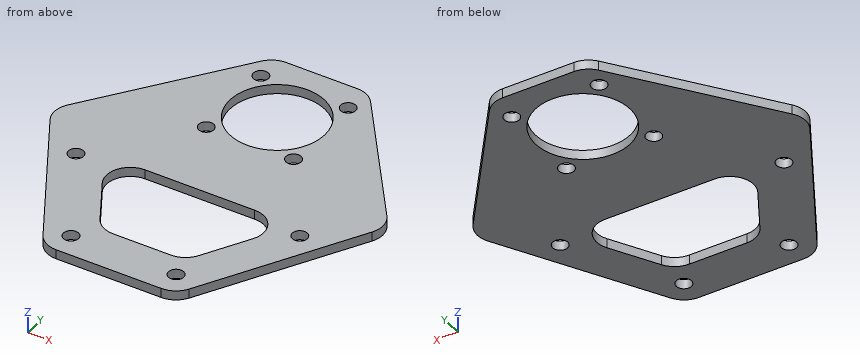
```python
from build123d import *

# Parameters (mm, degrees)
EXTRUDE_1_OUTLINE_R   = 1.6
EXTRUDE_1_OUTLINE_R_2 = 10
EXTRUDE_1_DEPTH       = 2
FILLET_1_R            = 5


# Read off the part's stored shape, not the designer's step: ﾎﾞｽ - 押し出し1
with BuildPart() as part:
    # ﾎﾞｽ - 押し出し1 outline → ﾎﾞｽ - 押し出し1 (new body)
    with BuildSketch(Plane.XY):
        Polygon((-15.011106999, -35), (12.897858345, -35), (34.473029949, 2.369293401), (10, 35), (-10, 35), (-35.667090423, 0.77721277), align=None)
        with Locations((-12.124355653, -30)):
            Circle(EXTRUDE_1_OUTLINE_R, mode=Mode.SUBTRACT)
        with Locations((-24.624355653, -8.349364905)):
            Circle(EXTRUDE_1_OUTLINE_R, mode=Mode.SUBTRACT)
        with Locations((10.011106999, -30)):
            Circle(EXTRUDE_1_OUTLINE_R, mode=Mode.SUBTRACT)
        with BuildLine():
            Line((6.062177826, -25.5), (-6.062177826, -25.5))
            ThreePointArc((-6.062177826, -25.5), (-8.562177826, -24.830127019), (-10.392304845, -23))
            Line((-10.392304845, -23), (-15.877132403, -13.5))
            ThreePointArc((-15.877132403, -13.5), (-15.877132403, -8.5), (-11.547005384, -6))
            Line((-11.547005384, -6), (11.547005384, -6))
            ThreePointArc((11.547005384, -6), (15.877132403, -8.5), (15.877132403, -13.5))
            Line((15.877132403, -13.5), (10.392304845, -23))
            ThreePointArc((10.392304845, -23), (8.562177826, -24.830127019), (6.062177826, -25.5))
        make_face(mode=Mode.SUBTRACT)
        with Locations((22.511106999, -8.349364905)):
            Circle(EXTRUDE_1_OUTLINE_R, mode=Mode.SUBTRACT)
        with Locations((-9.192388155, 10.807611845)):
            Circle(EXTRUDE_1_OUTLINE_R, mode=Mode.SUBTRACT)
        with Locations((-9.192388155, 29.192388155)):
            Circle(EXTRUDE_1_OUTLINE_R, mode=Mode.SUBTRACT)
        with Locations((9.192388155, 10.807611845)):
            Circle(EXTRUDE_1_OUTLINE_R, mode=Mode.SUBTRACT)
        with Locations((0, 20)):
            Circle(EXTRUDE_1_OUTLINE_R_2, mode=Mode.SUBTRACT)
        with Locations((9.192388155, 29.192388155)):
            Circle(EXTRUDE_1_OUTLINE_R, mode=Mode.SUBTRACT)
    extrude(amount=EXTRUDE_1_DEPTH)

    # ﾌｨﾚｯﾄ1
    fillet_1_edges = [part.edges().sort_by_distance(p)[0] for p in [
        (12.897858345, -35, 1),
        (-15.011106999, -35, 1),
        (-35.667090423, 0.77721277, 1),
        (-10, 35, 1),
        (10, 35, 1),
        (34.473029949, 2.369293401, 1),
    ]]
    fillet(fillet_1_edges, radius=FILLET_1_R)


solid = part.part
```
Can you work these out from the model? Positions are in its coordinate system, mm. Give positions to 0.01 mm unless a question says otherwise; leave off trailing zeros. Write each loop counter-clockwise with the first axis right and the second up, starting at its lowest first coordinate (ties: lowest second). Pieces come first, ordered by that corner, then holes. Notation, with made-up numbers: (-20.75, 70.25) -> (37.25, 70.25) arc R16 cw to (37.25, 100.25) -> close; hole circle Ø1 at (-21.5, -37.5). An arc over 180 degrees is marked (long way). Write item = value, one per line.
(1) Suppose I cut it at D-D on y = -30. Write out the boundary of the cut face in (x, z).
Worked out:
outline = (-17.9, 0) -> (-13.72, 0) -> (-13.72, 2) -> (-17.9, 2) -> close; (-10.52, 0) -> (8.41, 0) -> (8.41, 2) -> (-10.52, 2) -> close; (11.61, 0) -> (15.78, 0) -> (15.78, 2) -> (11.61, 2) -> close
(2) Suppose I cut it at A-A on x = 0. Write out the boundary of the cut face in (y, z), then the cut area to 3 significant figures.
Worked out:
outline = (-35, 0) -> (-25.5, 0) -> (-25.5, 2) -> (-35, 2) -> close; (-6, 0) -> (10, 0) -> (10, 2) -> (-6, 2) -> close; (30, 0) -> (35, 0) -> (35, 2) -> (30, 2) -> close
area = 61.0 mm^2
(3) Suppose I cut it at C-C on z = 1.6. Count the separate pieces of the cut face and the enclosed holes in it, then the cut area to 3 significant figures.
Worked out:
separate_pieces = 1
enclosed_holes = 10
area = 2,380 mm^2
(4) I need wall thicknesses on probe 1 along X at (y, z) = (-8, 1.4); probe 2 along Y at (x, z) = (-11, 1.65); probe 3 along Y at (x, z) = (-8, 1.25). Which ranges of each line are inside material? Lowest first, please. Write a range as from..to.
Worked out:
probe_1 = -30.6..-26.19, -23.06..-15.55, 15.55..20.95, 24.07..28.49
probe_2 = -35..-31.14, -28.86..-21.95, -6..33.57
probe_3 = -35..-25.11, -6..9.74, 11.87..14, 26..28.13, 30.26..34.97
(5) Suppose I cut it at B-B on y = 20. Write out the boundary of the cut face in (x, z), then the cut area to 3 significant figures.
Worked out:
outline = (-21.25, 0) -> (-10, 0) -> (-10, 2) -> (-21.25, 2) -> close; (10, 0) -> (21.25, 0) -> (21.25, 2) -> (10, 2) -> close
area = 45.0 mm^2
